Source: CAD feature listing. Evaluate the final solid. Frame: model axes, mm. A direction names the side the tool comes from. Round coordinates to 2 decimals unless told otherwise and drop trailing zeros. Order: outer loops, then holes, each group sorted by start corner. A loop starts at its lowest first (then second) coordinate and runs counter-clockwise, first axis right, second up. Notation, with made-up numbers: M 13.5,-8.5 L 41.5,-8.5 A5 ccw 41.5,-1.5 Z; hole C 72.25,-28 d7. An arc over 180 degrees is marked long. Answer as CSV lines item,"result". Start each with the question number.
Item 1: Section query D-D on z = 16.5. Return the cut outline in (x, y), plus the area to 3 significant figures.
Item 2: Pull-direction query (Z, two-part tool) for faces 3 (the face through (-52.692, 2.348, 31.523)), 4 (the face through (89, 2, 0)), 5 (the face through (1, 0, -53)); classes: +Z half, -Z half, draft (parallel to the pull), parting line (faces both ways), or undercut.
Item 3: Section query C-C on y = 2.65. State how many separate pieces and enclosed holes the cut face has, plus the area to 3 significant figures.
Item 4: Line query: line 1 (X direction, y = 4.35, z = 27); line 2 (Z direction, x = -88.5, y = 3.85); line 3 (X direction, y = 1.9, z = -5.5). Output: solid intervals per line, ascending. Write a range as [from, to].
Item 5: Section query B-B on z = -24.5. Return the cut outline in (x, y), plus the area to 3 significant figures.
Item 6: Section query A-A on x = 0. Return the cut outline in (y, z).
Item 7: Set-up query: faces 1 (the face through (-101.6, 2, -50)), 2 (the face through (-89, 2, 0)). Return all of +Z, -Z, +X, -X, +Y, -Y with unobstructed straight access to the full face (end or side cutting, diameter ignored); none if empty.
from build123d import *

# Parameters (mm, degrees)
SKETCH1_R           = 3.175
SKETCH1_R_2         = 38.1
BOSS_EXTRUDE1_DEPTH = 4.7625


with BuildPart() as part:
    # Sketch1 → Boss-Extrude1 (new body)
    with BuildSketch(Plane(origin=(0, 0, 0), x_dir=(1, 0, 0), z_dir=(0, 1, 0))):
        with BuildLine():
            Line((-101.6, 0), (-101.6, 101.6))
            Line((-101.6, 101.6), (101.6, 101.6))
            Line((101.6, 101.6), (101.6, 0))
            Line((101.6, 0), (76.2, 0))
            ThreePointArc((76.2, 0), (0, -76.2), (-76.2, 0))
            Line((-76.2, 0), (-101.6, 0))
        make_face()
        with Locations(Location((0, 58.365493413, 0), (0, 0, 90))):
            Circle(SKETCH1_R, mode=Mode.SUBTRACT)
        with Locations(Location((-50.546, -29.182746706, 0), (0, 0, 90))):
            Circle(SKETCH1_R, mode=Mode.SUBTRACT)
        with Locations(Location((50.546, -29.182746706, 0), (0, 0, 90))):
            Circle(SKETCH1_R, mode=Mode.SUBTRACT)
        with Locations(Location((0, 0, 0), (0, 0, 90))):
            Circle(SKETCH1_R_2, mode=Mode.SUBTRACT)
    extrude(amount=BOSS_EXTRUDE1_DEPTH)


solid = part.part
Results:
1,outline,"M -74.39,0 L -34.34,0 L -34.34,4.76 L -74.39,4.76 Z; M 34.34,0 L 74.39,0 L 74.39,4.76 L 34.34,4.76 Z"
1,area,"381 mm^2"
2,face 3,"undercut"
2,face 4,"+Z half"
2,face 5,"draft"
3,separate pieces,"1"
3,enclosed holes,"4"
3,area,"25,100 mm^2"
4,line 1,"[-71.26, -52.85], [-48.24, -26.88], [26.88, 48.24], [52.85, 71.26]"
4,line 2,"[-101.6, 0]"
4,line 3,"[-101.6, -37.7], [37.7, 101.6]"
5,outline,"M -101.6,0 L -29.18,0 L -29.18,4.76 L -101.6,4.76 Z; M 29.18,0 L 101.6,0 L 101.6,4.76 L 29.18,4.76 Z"
5,area,"690 mm^2"
6,outline,"M 0,-101.6 L 4.76,-101.6 L 4.76,-61.54 L 0,-61.54 Z; M 0,-55.19 L 4.76,-55.19 L 4.76,-38.1 L 0,-38.1 Z; M 0,38.1 L 4.76,38.1 L 4.76,76.2 L 0,76.2 Z"
7,face 1,"+Z, -Z, -X, +Y, -Y"
7,face 2,"+Z, -X, +Y, -Y"
